CAD build for the part. Positions are in the model's coordinates, mm. Face numbers are marked on the shaded views. A direction names the side the tool comes from. Give positions to 0.01 mm unless a question says otherwise; leave off trailing zeros. Write each loop counter-clockwise with the first axis right and the second up, starting at its lowest first coordinate (ties: lowest second). Pieces come first, ordered by that corner, then holes. Notation, with made-up numbers: M 7,-5 L 66,-5 A15 cw 66,11 Z; hole C -10.5,86 d2. An arc over 180 degrees is marked long. One line per question, with ' | ' between items. Start each with the question number.
1. Cut at D-D, the plane y = 11.5. Count the separate pieces of the cut face and the enclosed holes in it, then the cut area to 3 significant figures.
2. Which spindle directions (+Z, -Z, +X, -X, +Y, -Y) get a long thin tool onto all of the face, cutting with end or side? Do the marked faces 4, 5 and 6. Say none if no direction does.
3. Cut at C-C, the plane x = 61.5. Write the cut outline in (y, z), then the cut area to 3 significant figures.
4. Cut at B-B, the plane z = -24. Write the cut outline in (x, y).
5. Cut at A-A, the plane x = 19. Write the cut outline in (y, z).
6. Wall check: L1, parallel to X at y = 42, z = -7; L2, parallel to Y at x = 59, z = -9.5; L3, parallel to Z at x = 5, y = 38.5. Give the ranges that are in metal, low to high.
7. Pull direction X, two halves, no side cores. Call the marked faces 1, 2 and 3: released by +X, released by -X, zero draft, split by the parting line, or undercut.
8. Flat gauge pins, fed straight in: pin 1 (3.5 mm diameter, centred on x = 81.5, z = -35, fed in from -Y); pin 2 (1.6 mm diameter, centred on x = 50.5, z = -1, fed in from -Y); pin 3 (1.6 mm diameter, centred on y = 18.5, z = -1, fed in from -X); pin 4 (10 mm diameter, centred on x = 13.5, y = 29.5, fed in from +Z). Where does each tip first touch, or does it go through?
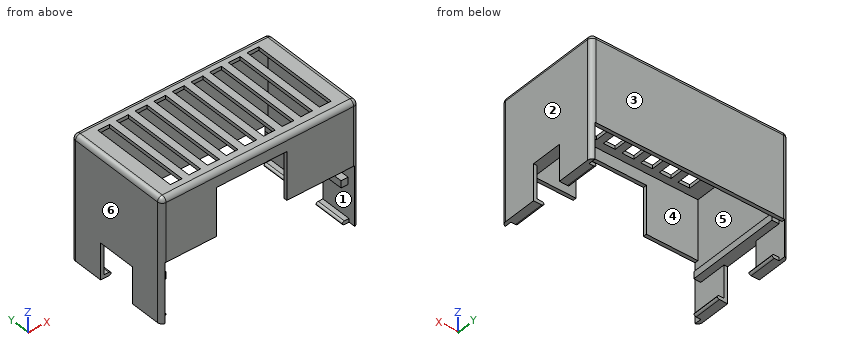
```python
from build123d import *

# Parameters (mm, degrees)
F0_W         = 84
F0_H         = 46.33
F1_DEPTH     = 37
F2_T         = -1.5
F4_W         = 81
F4_H         = 10
F5_DEPTH     = 1.5
F6_W         = 30
F6_H         = 20.5
F7_DEPTH     = 1.5
F9_DEPTH     = 15.5
F10_W        = 40.33
F10_H        = 3
F11_DEPTH    = 3
F12_W        = 39.33
F12_H        = 3
F13_DEPTH    = 3
F14_W        = 1.5
F14_H        = 13.33
F15_DEPTH    = 15.5
F16_W        = 1.5
F16_H        = 16.33
F17_DEPTH    = 15.5
F18_W        = 12
F18_H        = 1.5
F19_DEPTH    = 3
F20_W        = 13.5
F20_H        = 1.5
F21_DEPTH    = 3
F22_W        = 5
F22_H        = 37.33
F23_DEPTH    = 1.5
F24_R        = 2
F25_T1_DEPTH = 17
F25_T3_DEPTH = 17
F25_T5_DEPTH = 18.5
F25_T7_DEPTH = 18.5


# Not quite as in the source:
# - a fillet or chamfer that OpenCascade refuses, or shapes differently, is made with other operations: its cross-section is extruded or revolved along the edge and cut away or added


with BuildPart() as f1:
    # F0 (on Top) → F1 (new body)
    with BuildSketch(Plane.XY):
        with Locations((42, 23.165)):
            Rectangle(F0_W, F0_H)
    extrude(amount=-F1_DEPTH)

    # F2
    f2_openings = [f1.faces().sort_by_distance(p)[0] for p in [
        (42, 23.165, -37),
    ]]
    offset(amount=F2_T, openings=f2_openings)

    # F4 (on face) → F5 (cut, through all)
    with BuildSketch(Plane.XZ):
        with Locations((42, -32)):
            Rectangle(F4_W, F4_H)
    extrude(amount=-F5_DEPTH, mode=Mode.SUBTRACT)

    # F6 (on face) → F7 (cut, through all)
    with BuildSketch(Plane.XZ):
        with Locations((38.5, -16.75)):
            Rectangle(F6_W, F6_H)
    extrude(amount=-F7_DEPTH, mode=Mode.SUBTRACT)

    # F8 (on face) → F9 (join)
    with BuildSketch(Plane(origin=(0, 0, -37), x_dir=(1, 0, 0), z_dir=(0, 0, -1))):
        Polygon((0, 0), (0, -46.33), (1.5, -46.33), (1.5, -44.83), (1.5, 0), align=None)
        Polygon((82.5, -44.83), (82.5, -46.33), (84, -46.33), (84, 0), (82.5, 0), align=None)
    extrude(amount=F9_DEPTH)

    # F10 (on face) → F11 (join)
    with BuildSketch(Plane.YZ.offset(1.5)):
        with Locations((23.165, -35.5)):
            Rectangle(F10_W, F10_H)
    extrude(amount=F11_DEPTH)

    # F12 (on face) → F13 (join)
    with BuildSketch(Plane(origin=(82.5, 0, 0), x_dir=(0, -1, 0), z_dir=(-1, 0, 0))):
        with Locations((-23.165, -35.5)):
            Rectangle(F12_W, F12_H)
    extrude(amount=F13_DEPTH)

    # F14 (on face) → F15 (cut)
    with BuildSketch(Plane(origin=(0, 0, -52.5), x_dir=(1, 0, 0), z_dir=(0, 0, -1))):
        with Locations((83.25, -23.165)):
            Rectangle(F14_W, F14_H)
    extrude(amount=-F15_DEPTH, mode=Mode.SUBTRACT)

    # F16 (on face) → F17 (cut)
    with BuildSketch(Plane(origin=(0, 0, -52.5), x_dir=(1, 0, 0), z_dir=(0, 0, -1))):
        with Locations((0.75, -23.165)):
            Rectangle(F16_W, F16_H)
    extrude(amount=-F17_DEPTH, mode=Mode.SUBTRACT)

    # F18 (on face) → F19 (join)
    with BuildSketch(Plane.YZ.offset(1.5)):
        with Locations((37.33, -51.75)):
            Rectangle(F18_W, F18_H)
        with Locations((9, -51.75)):
            Rectangle(F18_W, F18_H)
    extrude(amount=F19_DEPTH)

    # F20 (on face) → F21 (join)
    with BuildSketch(Plane(origin=(82.5, 0, 0), x_dir=(0, -1, 0), z_dir=(-1, 0, 0))):
        with Locations((-9.75, -51.75)):
            Rectangle(F20_W, F20_H)
        with Locations((-36.58, -51.75)):
            Rectangle(F20_W, F20_H)
    extrude(amount=F21_DEPTH)

    # F22 (on face) → F23 (cut, through all)
    with BuildSketch(Plane(origin=(0, 0, -1.5), x_dir=(1, 0, 0), z_dir=(0, 0, -1))):
        with Locations((73.9982255152, -23.6415825304)):
            Rectangle(F22_W, F22_H)
        with Locations((65.9984473258, -23.5820097141)):
            Rectangle(F22_W, F22_H)
        with Locations((49.998890947, -23.4628640815)):
            Rectangle(F22_W, F22_H)
        with Locations((41.9991127576, -23.4032912652)):
            Rectangle(F22_W, F22_H)
        with Locations((33.9993345682, -23.3437184489)):
            Rectangle(F22_W, F22_H)
        with Locations((25.9995563788, -23.2841456326)):
            Rectangle(F22_W, F22_H)
        with Locations((17.9997781894, -23.2245728163)):
            Rectangle(F22_W, F22_H)
        with Locations((10, -23.165)):
            Rectangle(F22_W, F22_H)
        with Locations((57.9986691364, -23.5224368978)):
            Rectangle(F22_W, F22_H)
    extrude(amount=-F23_DEPTH, mode=Mode.SUBTRACT)

    # F24
    f24_edges = [f1.edges().sort_by_distance(p)[0] for p in [
        (42, 0, 0),
        (84, 23.165, 0),
        (84, 0, -26.25),
        (84, 46.33, -26.25),
        (42, 46.33, 0),
        (0, 46.33, -26.25),
        (0, 23.165, 0),
        (0, 0, -26.25),
    ]]
    fillet(f24_edges, radius=F24_R)

    # F25: fillet of radius 1 on 8 edges, made by hand

    # F25_s2 → F25_t1 (cut)
    with BuildSketch(Plane.XZ.offset(-17.5)):
        with BuildLine():
            ThreePointArc((3.5, -52.5), (4.2071067812, -52.2071067812), (4.5, -51.5))
            Line((4.5, -51.5), (4.5, -52.5))
            Line((4.5, -52.5), (3.5, -52.5))
        make_face()
        with BuildLine():
            ThreePointArc((4.5, -52), (4.2071067812, -51.2928932188), (3.5, -51))
            Line((3.5, -51), (4.5, -51))
            Line((4.5, -51), (4.5, -52))
        make_face()
    extrude(amount=F25_T1_DEPTH, mode=Mode.SUBTRACT)

    # F25_s4 → F25_t3 (cut)
    with BuildSketch(Plane.XZ.offset(-45.83)):
        with BuildLine():
            ThreePointArc((3.5, -52.5), (4.2071067812, -52.2071067812), (4.5, -51.5))
            Line((4.5, -51.5), (4.5, -52.5))
            Line((4.5, -52.5), (3.5, -52.5))
        make_face()
        with BuildLine():
            ThreePointArc((3.5, -51), (4.2071067812, -51.2928932188), (4.5, -52))
            Line((4.5, -52), (4.5, -51))
            Line((4.5, -51), (3.5, -51))
        make_face()
    extrude(amount=F25_T3_DEPTH, mode=Mode.SUBTRACT)

    # F25_s6 → F25_t5 (cut)
    with BuildSketch(Plane.XZ.offset(-19)):
        with BuildLine():
            ThreePointArc((80.5, -51), (79.7928932188, -51.2928932188), (79.5, -52))
            Line((79.5, -52), (79.5, -51))
            Line((79.5, -51), (80.5, -51))
        make_face()
        with BuildLine():
            ThreePointArc((80.5, -52.5), (79.7928932188, -52.2071067812), (79.5, -51.5))
            Line((79.5, -51.5), (79.5, -52.5))
            Line((79.5, -52.5), (80.5, -52.5))
        make_face()
    extrude(amount=F25_T5_DEPTH, mode=Mode.SUBTRACT)

    # F25_s8 → F25_t7 (cut)
    with BuildSketch(Plane.XZ.offset(-45.83)):
        with BuildLine():
            ThreePointArc((80.5, -52.5), (79.7928932188, -52.2071067812), (79.5, -51.5))
            Line((79.5, -51.5), (79.5, -52.5))
            Line((79.5, -52.5), (80.5, -52.5))
        make_face()
        with BuildLine():
            ThreePointArc((80.5, -51), (79.7928932188, -51.2928932188), (79.5, -52))
            Line((79.5, -52), (79.5, -51))
            Line((79.5, -51), (80.5, -51))
        make_face()
    extrude(amount=F25_T7_DEPTH, mode=Mode.SUBTRACT)


solid = f1.part
```
Here are the results:
1) separate pieces: 10 | enclosed holes: 0 | area: 236 mm^2
2) face 4: -Z | face 5: none | face 6: +Z, -Z, -X, +Y, -Y
3) outline: M 0,-27 L 1.5,-27 L 1.5,-1.5 L 44.83,-1.5 L 44.83,-37 L 46.33,-37 L 46.33,-2 A2 ccw 44.33,0 L 2,0 A2 ccw 0,-2 Z | area: 159 mm^2
4) outline: M 0,2 A2 ccw 2,0 L 23.5,0 L 23.5,1.5 L 1.5,1.5 L 1.5,44.83 L 82.5,44.83 L 82.5,1.5 L 53.5,1.5 L 53.5,0 L 82,0 A2 ccw 84,2 L 84,44.33 A2 ccw 82,46.33 L 2,46.33 A2 ccw 0,44.33 Z
5) outline: M 0,-27 L 1.5,-27 L 1.5,-1.5 L 4.56,-1.5 L 4.56,0 L 2,0 A2 ccw 0,-2 Z; M 41.89,-1.5 L 44.83,-1.5 L 44.83,-37 L 46.33,-37 L 46.33,-2 A2 ccw 44.33,0 L 41.89,0 Z
6) L1: 0 to 1.5, 82.5 to 84 | L2: 0 to 1.5, 44.83 to 46.33 | L3: -1.5 to 0
7) face 1: undercut | face 2: released by +X | face 3: zero draft
8) pin 1: y = 0.06 | pin 2: y = 0.01 | pin 3: x = 0.01 | pin 4: z = 0
